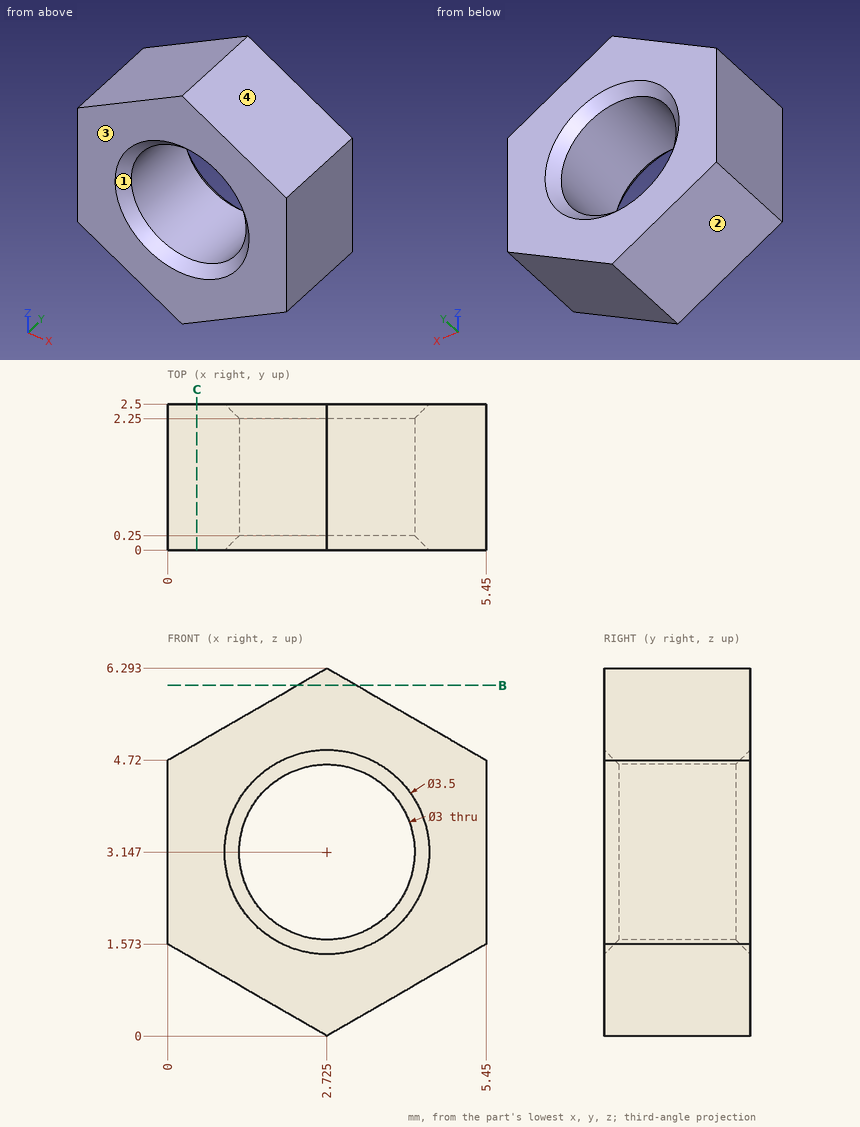
Study the drawing (mm; zero at the part's minimum x, y, z) and answer. Give positions to 0.01 mm unless a question says otherwise; leave off trailing zeros. Order: outer loops, then holes, each group sorted by start corner. A loop starts at its lowest first (then second) coordinate and runs counter-clockwise, first axis right, second up. Notation, with made-up numbers: M 11.25,-17.75 L 57.25,-17.75 A19 cw 57.25,-5.75 Z; hole C 64,64.25 d3. An arc over 180 degrees is marked long. Put each result on its own line as item: value. Start each with the question number.
Item 1: Find the intervals of material crossed by line 1 along Z through (x, y) = (3, 2.35) (1 decimal); line 2 along Z through (x, y) = (1.9, 1.4) (1 decimal); line 3 along X through (y, z) = (1.6, 4), in increasing order.
Item 2: The part is cut by section B-B, the plane z = 6. Determine the outline of the cut face in (x, y).
Item 3: For a pull along Z with two mould halves and no side action, classify the marked faces 1, 2, 3 and 4 as +Z half, -Z half, draft (parallel to the pull), parting line (faces both ways), or undercut.
Item 4: The part is cut by section C-C, the plane x = 0.5. Determine the outline of the cut face in (y, z) (1 decimal).
Answer key:
1. line 1: z = 0.2 to 1.6, 4.7 to 6.1
1. line 2: z = 0.5 to 1.9, 4.4 to 5.8
1. line 3: x = 0 to 1.49, 3.96 to 5.45
2. outline: M 2.22,0 L 3.23,0 L 3.23,2.5 L 2.22,2.5 Z
3. face 1: undercut
3. face 2: -Z half
3. face 3: draft
3. face 4: +Z half
4. outline: M 0,1.3 L 2.5,1.3 L 2.5,5 L 0,5 Z
